```python
from build123d import *

# Parameters (mm, degrees)
SKETCH_1_R               = 12
SKETCH_1_R_2             = 9.25
EXTRUDE_1_DEPTH          = 30
EXTRUDE_2_REACH          = 86.467
EXTRUDE_2_END_RADIUS     = 12
EXTRUDE_START            = 50
SKETCH_2_R               = 12
SKETCH_2_R_2             = 9.25
SKETCH_3_R               = 1.75
CUT_EXTRUDE_1_DEPTH      = 60.531504349
CUT_EXTRUDE_1_DEPTH_BACK = 60.531504349
SKETCH_4_R               = 1.75
CUT_EXTRUDE_2_DEPTH      = 60.531504419
CUT_EXTRUDE_2_DEPTH_BACK = 60.531504419
EXTRUDE_3_DEPTH          = 2.5
CUT_EXTRUDE_3_REACH      = 71.914
SKETCH_6_R               = 9.25


with BuildPart() as part:
    # Sketch 1 → Extrude 1 (new, symmetric)
    with BuildSketch(Plane(origin=(0, 0, 0), x_dir=(1, 0, 0), z_dir=(0, 1, 0))):
        with Locations(Location((0, 0, 0), (0, 0, 270))):
            Circle(SKETCH_1_R)
        with Locations(Location((0, 0, 0), (0, 0, 270))):
            Circle(SKETCH_1_R_2, mode=Mode.SUBTRACT)
    extrude(amount=EXTRUDE_1_DEPTH, both=True)

    # Extrude 2: up to this cylinder (the profile starts outside it)
    extrude_2_end = Plane(origin=(0, 0, 0), z_dir=(0, -1, 0)) * Cylinder(EXTRUDE_2_END_RADIUS, 197.934, mode=Mode.PRIVATE)
    # Sketch 2 → Extrude 2 (add, up to the surface)
    with BuildSketch(Plane(origin=(0, 0, 0), x_dir=(0, 0, -1), z_dir=(1, 0, 0)).offset(EXTRUDE_START), mode=Mode.PRIVATE) as extrude_2_sk1:
        Circle(SKETCH_2_R)
        Circle(SKETCH_2_R_2, mode=Mode.SUBTRACT)
    extrude_2_tool1 = extrude(extrude_2_sk1.sketch, amount=-EXTRUDE_2_REACH, mode=Mode.PRIVATE) - extrude_2_end
    add(extrude_2_tool1.solids().sort_by_distance((50, 0, 11.660589))[0])

    # Sketch 3 → Cut-Extrude 1 (cut, two sides)
    with BuildSketch(Plane(origin=(0, 0, 0), x_dir=(0, -1, 0), z_dir=(0.499999999999998, 0, 0.8660254037844398))) as cut_extrude_1_sk:
        with Locations(Location((-20, 0, 0), (0, 0, 90))):
            Circle(SKETCH_3_R)
        with Locations(Location((20, 0, 0), (0, 0, 90))):
            Circle(SKETCH_3_R)
    extrude(amount=CUT_EXTRUDE_1_DEPTH, mode=Mode.SUBTRACT)
    extrude(cut_extrude_1_sk.sketch, amount=-CUT_EXTRUDE_1_DEPTH_BACK, mode=Mode.SUBTRACT)

    # Sketch 4 → Cut-Extrude 2 (cut, two sides)
    with BuildSketch(Plane.XY) as cut_extrude_2_sk:
        with Locations((20, 0)):
            Circle(SKETCH_4_R)
        with Locations((40, 0)):
            Circle(SKETCH_4_R)
    extrude(amount=CUT_EXTRUDE_2_DEPTH, mode=Mode.SUBTRACT)
    extrude(cut_extrude_2_sk.sketch, amount=-CUT_EXTRUDE_2_DEPTH_BACK, mode=Mode.SUBTRACT)

    # Sketch 5 → Extrude 3 (add, symmetric)
    with BuildSketch(Plane.XY):
        Polygon((10.496083989, 27.069423811), (33.248789053, 10.881728509), (10.496083989, 10.496083989), align=None)
        Polygon((33.248789053, -10.881728509), (10.496083989, -10.496083989), (10.496083989, -27.069423811), align=None)
    extrude(amount=EXTRUDE_3_DEPTH, both=True)

    # Sketch 6 → Cut-Extrude 3 (cut, up to next)
    with BuildSketch(Plane(origin=(50, 0, 0), x_dir=(0, 0, -1), z_dir=(1, 0, 0)), mode=Mode.PRIVATE) as cut_extrude_3_sk1:
        Circle(SKETCH_6_R)
    cut_extrude_3_tool1 = extrude(cut_extrude_3_sk1.sketch, amount=-CUT_EXTRUDE_3_REACH, mode=Mode.PRIVATE) & part.part
    add(cut_extrude_3_tool1.solids().sort_by_distance((50, 0, 0))[0], mode=Mode.SUBTRACT)


solid = part.part
```
Read the model definition and answer for the solid it produces. Units are mm, in the model's axes. A direction names the side the tool comes from. Coordinates: 2 decimals unless noted, no trailing zeros. Write each loop counter-clockwise with the first axis right and the second up, starting at its lowest first coordinate (ties: lowest second). Pieces come first, ordered by that corner, then holes. Notation, with made-up numbers: (43.25, 47.5) -> (85.25, 47.5) arc R20 cw to (85.25, 58.5) -> close; hole circle Ø7 at (47.5, -28.75). An arc over 180 degrees is marked (long way). Return JSON: item names as keys, results as strings.
1. A cutting plane is placed at B-B (z = 0). Determine the outline of the cut face in (x, y), and give its area (3 significant figures).
Found:
{"outline": "(-12, -30) -> (-9.25, -30) -> (-9.25, 30) -> (-12, 30) -> close; (9.25, -30) -> (12, -30) -> (12, -26) -> (31.68, -12) -> (50, -12) -> (50, -9.25) -> (9.25, -9.25) -> close; (9.25, 9.25) -> (50, 9.25) -> (50, 12) -> (31.68, 12) -> (12, 26) -> (12, 30) -> (9.25, 30) -> close", "area": "764 mm2"}
2. A tool of negligible diameter and unlimited length cuts with its end or side. For faces 1 (the face through (30.906, -10.646, -5.537)), 2 (the face through (18, 16, 2.5)), 3 (the face through (18, 16, -2.5)), from which of +Z, -Z, +X, -X, +Y, -Y can it reach the whole face along a straight path? Write none if from no direction.
Found:
{"face 1": "+X", "face 2": "+Z, +X, +Y", "face 3": "-Z, +X, +Y"}
3. A cutting plane is placed at C-C (y = 10). Determine the outline of the cut face in (x, z), and give its area (3 significant figures).
Found:
{"outline": "(10, -6.63) -> (50, -6.63) -> (50, 6.63) -> (10, 6.63) arc R12 ccw (long way) to start; hole circle Ø18.5 at (0, 0)", "area": "696 mm2"}
4. Determine the mould class of faces 4 (the face through (-3.815, 20.526, -9.946)), 5 (the face through (21.7, 19.1, 0)), 6 (the face through (-3.815, -19.474, -9.946)), 7 (the face through (19, -17, -2.5)) for opening direction Z: pulls with the +Z half, pulls with the -Z half, needs draft (parallel to the pull), parting line crosses it, or undercut.
Found:
{"face 4": "undercut", "face 5": "needs draft", "face 6": "undercut", "face 7": "pulls with the -Z half"}
5. Find the intervals of material crossed by line 1 along Z through (x, y) = (-0.5, -24.5); line 2 along X through (y, z) = (0, -9.8); line 3 along Y through (x, z) = (8, -6.5), in increasing order. Write a range as from..to.
Found:
{"line 1": "-11.99..-9.24, 9.24..11.99", "line 2": "-6.93..18.25, 21.75..38.25, 41.75..50", "line 3": "-30..-6.58, 6.58..30"}
6. A cutting plane is placed at A-A (y = 0). Determine the outline of the cut face in (x, z), and give its area (3 significant figures).
Found:
{"outline": "(0, -12) -> (18.25, -12) -> (18.25, -9.25) -> (0, -9.25) arc R9.25 cw to (0, 9.25) -> (18.25, 9.25) -> (18.25, 12) -> (0, 12) arc R12 ccw to start; (21.75, -12) -> (38.25, -12) -> (38.25, -9.25) -> (21.75, -9.25) -> close; (21.75, 9.25) -> (38.25, 9.25) -> (38.25, 12) -> (21.75, 12) -> close; (41.75, -12) -> (50, -12) -> (50, -9.25) -> (41.75, -9.25) -> close; (41.75, 9.25) -> (50, 9.25) -> (50, 12) -> (41.75, 12) -> close", "area": "328 mm2"}
7. Each of these flat-tipped pins is pushed along its axis until it touches: P1, Ø11.5, axis at x = 21.5, y = 18, coming from the -Z side; P2, Ø16, axis at x = 26, y = -18, coming from the +Z side; P3, Ø10, axis at y = -6.5, z = 5.5, coming from the +X side; P4, Ø3, axis at x = 40, y = 0, coming from the -Z side. Where does it stop, or does it pass through?
Found:
{"P1": "z = -2.5", "P2": "z = 6.63", "P3": "x = 50", "P4": "through"}
8. A cutting plane is placed at D-D (z = 4.5). Determine the outline of the cut face in (x, y), and give its area (3 significant figures).
Found:
{"outline": "(-11.12, -30) -> (-8.08, -30) -> (-8.08, 30) -> (-11.12, 30) -> close; (8.08, -30) -> (11.12, -30) -> (11.12, -11.12) -> (50, -11.12) -> (50, -8.08) -> (8.08, -8.08) -> close; (8.08, 8.08) -> (50, 8.08) -> (50, 11.12) -> (11.12, 11.12) -> (11.12, 30) -> (8.08, 30) -> close", "area": "553 mm2"}
